from build123d import *

# Parameters (mm, degrees)
SKETCH1_W                  = 85
SKETCH1_H                  = 60
EXTRUDE1_DEPTH             = 15
F_12_0_12_DIAMETER_HOLE1_D = 12
SKETCH4_W                  = 37
SKETCH4_H                  = 30
CUT_EXTRUDE1_DEPTH         = 82.853527719
F_8_0_8_DIAMETER_HOLE1_D   = 8


with BuildPart() as part:
    # Sketch1 → Extrude1 (new, symmetric)
    with BuildSketch(Plane(origin=(0, 0, 0), x_dir=(1, 0, 0), z_dir=(0, 1, 0))):
        with Locations((-27.5, 0)):
            Rectangle(SKETCH1_W, SKETCH1_H)
    extrude(amount=EXTRUDE1_DEPTH, both=True)

    # Ø12.0 (12) Diameter Hole1 (through all)
    with Locations(Plane.XY.offset(30)):
        with Locations((0, 0)):
            Hole(F_12_0_12_DIAMETER_HOLE1_D / 2)

    # Sketch4 → Cut-Extrude1 (cut, through all)
    with BuildSketch(Plane(origin=(0, 15, 0), x_dir=(1, 0, 0), z_dir=(0, 1, 0))):
        with Locations((-3.5, 0)):
            Rectangle(SKETCH4_W, SKETCH4_H)
    extrude(amount=-CUT_EXTRUDE1_DEPTH, mode=Mode.SUBTRACT)

    # Ø8.0 (8) Diameter Hole1 (through all)
    with Locations(Plane.ZY.offset(70)):
        with Locations((0, 0)):
            Hole(F_8_0_8_DIAMETER_HOLE1_D / 2)

    # Sketch9 → M12x1.75 Tapped Hole1 (revolve, cut)
    with BuildSketch(Plane(origin=(-70, 0, -20), x_dir=(0, 0, 1), z_dir=(0, 1, 0))):
        Polygon((0, 0), (0, 30.314389157), (5.1, 27.25), (5.1, 0), align=None)
    m12x1_75_tapped_hole1 = revolve(axis=Axis((-76.35, 0, -20), (1, 0, 0)), mode=Mode.SUBTRACT)

    # Mirror1: M12x1.75 Tapped Hole1 across plane
    add(m12x1_75_tapped_hole1.mirror(Plane.XY), mode=Mode.SUBTRACT)


solid = part.part
Verification items for the finished model (mm, model axes). A direction names the side the tool comes from. Round coordinates to 2 decimals unless told otherwise and drop trailing zeros. Loops run counter-clockwise (first coordinate to the right, second up) from the corner with the lowest first, then second, coordinate; pieces in that order, holes last. Notation, with made-up numbers: (-6, -4) - (39, -4) arc R13 cw to (39, 10) - close; hole circle Ø3 at (61.25, 83.25). An arc over 180 degrees is marked (long way). Use a Markdown table: item, result. Add a question column.
1. Section check D-D, the plane y = -12. Record the boundary of the cut face in (x, z).
2. Release check for a two-part mould opening along X. For faces 1 (the face through (6, 0, -23)), 2 (the face through (15, 0, 23)), 3 (the face through (-38, 15, 0)) record: released by +X, released by -X, zero draft, split by the parting line, or undercut.
3. Section check A-A, the plane x = -17. Record the boundary of the cut face in (y, z), plus the area to 3 significant figures.
4. Access from +Z, -Z, +X, -X, +Y, -Y to the whole of each face (thin tool, end or side, straight path). Record for faces 4 (the face through (-38, -15, 0)), 5 (the face through (-56.57, 3.1, 24.05)), 6 (the face through (-8, 0, 15)).
5. Section check B-B, the plane x = 0. Record the boundary of the cut face in (y, z), plus the area to 3 significant figures.
6. Thickness scan on probe 1 along Z at (x, y) = (-19, 7.75); probe 2 along Y at (x, z) = (-50, 0); probe 3 along Y at (x, z) = (0, 24). Record the ranges inside material, lowest first. Write a range as [from, to].
7. Gauge pin test, flat ends, axial feed: pin 1 (9 mm diameter, centred on y = 0, z = 20, fed in from -X); pin 2 (15 mm diameter, centred on y = -7, z = 0.5, fed in from +X); pin 3 (14 mm diameter, centred on x = 0, y = 0, fed in from +Z). Record the tip position at first contact, or that the pin passes through.
8. Section check C-C, the plane z = 0. Record the boundary of the cut face in (x, y).
Checks:
| question | item | result |
|---|---|---|
| 1 | outline | (-70, -30) - (15, -30) - (15, -15) - (-22, -15) - (-22, 15) - (15, 15) - (15, 30) - (-70, 30) - close |
| 2 | face 1 | undercut |
| 2 | face 2 | released by +X |
| 2 | face 3 | zero draft |
| 3 | outline | (-15, -30) - (15, -30) - (15, -15) - (-15, -15) - close; (-15, 15) - (15, 15) - (15, 30) - (-15, 30) - close |
| 3 | area | 900 mm^2 |
| 4 | face 4 | +Z, -Z, +X, -X, -Y |
| 4 | face 5 | -X |
| 4 | face 6 | +X, +Y, -Y |
| 5 | outline | (-15, -30) - (-6, -30) - (-6, -15) - (-15, -15) - close; (-15, 15) - (-6, 15) - (-6, 30) - (-15, 30) - close; (6, -30) - (15, -30) - (15, -15) - (6, -15) - close; (6, 15) - (15, 15) - (15, 30) - (6, 30) - close |
| 5 | area | 540 mm^2 |
| 6 | probe 1 | z = [-30, -15], [15, 30] |
| 6 | probe 2 | y = [-15, -4], [4, 15] |
| 6 | probe 3 | y = [-15, -6], [6, 15] |
| 7 | pin 1 | stops at x = -42.39 |
| 7 | pin 2 | stops at x = -22 |
| 7 | pin 3 | stops at z = 30 |
| 8 | outline | (-70, -15) - (-22, -15) - (-22, -4) - (-70, -4) - close; (-70, 4) - (-22, 4) - (-22, 15) - (-70, 15) - close |
